Read the model definition and answer for the solid it produces. Units are mm, in the model's axes. A direction names the side the tool comes from. Coordinates: 2 decimals unless noted, no trailing zeros. Loops run counter-clockwise (first coordinate to the right, second up) from the corner with the lowest first, then second, coordinate; pieces in that order, holes last.
from build123d import *

# Parameters (mm, degrees)
SKETCH_1_R          = 5
EXTRUDE_1_DEPTH     = 10
FILLET_1_R          = 0.5
SKETCH_3_R          = 12.5
CUT_EXTRUDE_1_DEPTH = 6


with BuildPart() as part:
    # 草图1 → 凸台-拉伸1 (new, symmetric)
    with BuildSketch(Plane.XY):
        with BuildLine():
            Line((6.360983408, 12.421966817), (10, 4.5))
            Line((10, 4.5), (10, -4.5))
            Line((10, -4.5), (-10, -4.5))
            Line((-10, -4.5), (-10, 4.5))
            Line((-10, 4.5), (-6.360983408, 12.421966817))
            ThreePointArc((-6.360983408, 12.421966817), (0, 16.5), (6.360983408, 12.421966817))
        make_face()
        with Locations((0, 9.5)):
            Circle(SKETCH_1_R, mode=Mode.SUBTRACT)
    extrude(amount=EXTRUDE_1_DEPTH, both=True)

    # 圆角1
    fillet_1_edges = [part.edges().sort_by_distance(p)[0] for p in [
        (10, -4.5, 0),
        (-10, -4.5, 0),
        (-10, 4.5, 0),
        (10, 4.5, 0),
        (0, 16.5, 10),
        (-8.180491704, 8.460983408, 10),
        (-10, 0, 10),
        (0, -4.5, 10),
        (10, 0, 10),
        (0, -4.5, -10),
        (-10, 0, -10),
        (-8.180491704, 8.460983408, -10),
        (0, 16.5, -10),
        (8.180491704, 8.460983408, -10),
        (10, 0, -10),
        (8.180491704, 8.460983408, 10),
    ]]
    fillet(fillet_1_edges, radius=FILLET_1_R)

    # 草图3 → 切除-拉伸1 (cut, symmetric)
    with BuildSketch(Plane.XY):
        with Locations((0, 9.5)):
            Circle(SKETCH_3_R)
    extrude(amount=CUT_EXTRUDE_1_DEPTH, both=True, mode=Mode.SUBTRACT)


solid = part.part
Item 1: Given pin 1 (4 mm diameter, centred on x = -4.5, z = -6.5, fed in from +Y); pin 2 (10 mm diameter, centred on x = 1.5, y = 6.5, fed in from +Z); pin 3 (2 mm diameter, centred on y = 9, z = 3.5, fed in from -X); pin 4 (2 mm diameter, centred on x = -3, z = 2, fed in from +Y), each flat-ended and moving along its own axis, determine where each tip first touches the part or whether it passes through.
Numbers:
pin 1: stops at y = 16.04
pin 2: stops at z = 10
pin 3: passes through
pin 4: stops at y = -2.34
Item 2: Find the intervals of material crossed by line 1 along Z through (x, y) = (6.75, 7.5); line 2 along Y through (x, z) = (0, 8.85); line 3 along X through (y, z) = (9.5, 7.8), in increasing order.
Numbers:
line 1: z = -10 to -6, 6 to 10
line 2: y = -4.5 to 4.5, 14.5 to 16.5
line 3: x = -7.7 to -5, 5 to 7.7
Item 3: Determine the mould class of faces 3 (the face through (2.1, 4.7, 6)), 4 (the face through (8.1, 8.4, -9.8)), 5 (the face through (0, 4, -10)), 6 (the face through (2.1, 4.7, -6)) for opening direction X: released by +X, released by -X, zero draft, split by the parting line, or undercut.
Numbers:
face 3: undercut
face 4: released by +X
face 5: zero draft
face 6: undercut
Item 4: A cutting plane is placed at D-D on y = -1. Determine the outline of the cut face in (x, z), then the cut area to 3 significant figures.
Numbers:
outline: (-10, -9.5) arc R0.5 ccw to (-9.5, -10) - (9.5, -10) arc R0.5 ccw to (10, -9.5) - (10, 9.5) arc R0.5 ccw to (9.5, 10) - (-9.5, 10) arc R0.5 ccw to (-10, 9.5) - close; hole (-6.78, -6) - (6.78, -6) - (6.78, 6) - (-6.78, 6) - close
area: 237 mm2
Item 5: A cutting plane is placed at B-B on x = 0. Determine the outline of the cut face in (y, z), then the cut area to 3 significant figures.
Numbers:
outline: (-4.5, -9.5) arc R0.5 ccw to (-4, -10) - (4.5, -10) - (4.5, -6) - (-3, -6) - (-3, 6) - (4.5, 6) - (4.5, 10) - (-4, 10) arc R0.5 ccw to (-4.5, 9.5) - close; (14.5, -10) - (16, -10) arc R0.5 ccw to (16.5, -9.5) - (16.5, -6) - (14.5, -6) - close; (14.5, 6) - (16.5, 6) - (16.5, 9.5) arc R0.5 ccw to (16, 10) - (14.5, 10) - close
area: 106 mm2
Item 6: Which of the six approach directions +Z, -Z, +X, -X, +Y, -Y give full straight-line access (tool end or side, diameter ignored) to faces 1 (the face through (0, -3, 0)), 2 (the face through (-0.651, 14.457, -8.028))?
Numbers:
face 1: +Y
face 2: +Z, -Z
Item 7: A cutting plane is placed at C-C on z = 2.25. Determine the outline of the cut face in (x, y).
Numbers:
outline: (-10, -4) arc R0.5 ccw to (-9.5, -4.5) - (9.5, -4.5) arc R0.5 ccw to (10, -4) - (10, 2) arc R12.5 cw to (-10, 2) - close
Item 8: A cutting plane is placed at A-A on y = 2.5. Determine the outline of the cut face in (x, z), then the cut area to 3 significant figures.
Numbers:
outline: (-10, -9.5) arc R0.5 ccw to (-9.5, -10) - (9.5, -10) arc R0.5 ccw to (10, -9.5) - (10, -6) - (-10, -6) - close; (-10, 6) - (10, 6) - (10, 9.5) arc R0.5 ccw to (9.5, 10) - (-9.5, 10) arc R0.5 ccw to (-10, 9.5) - close
area: 160 mm2
